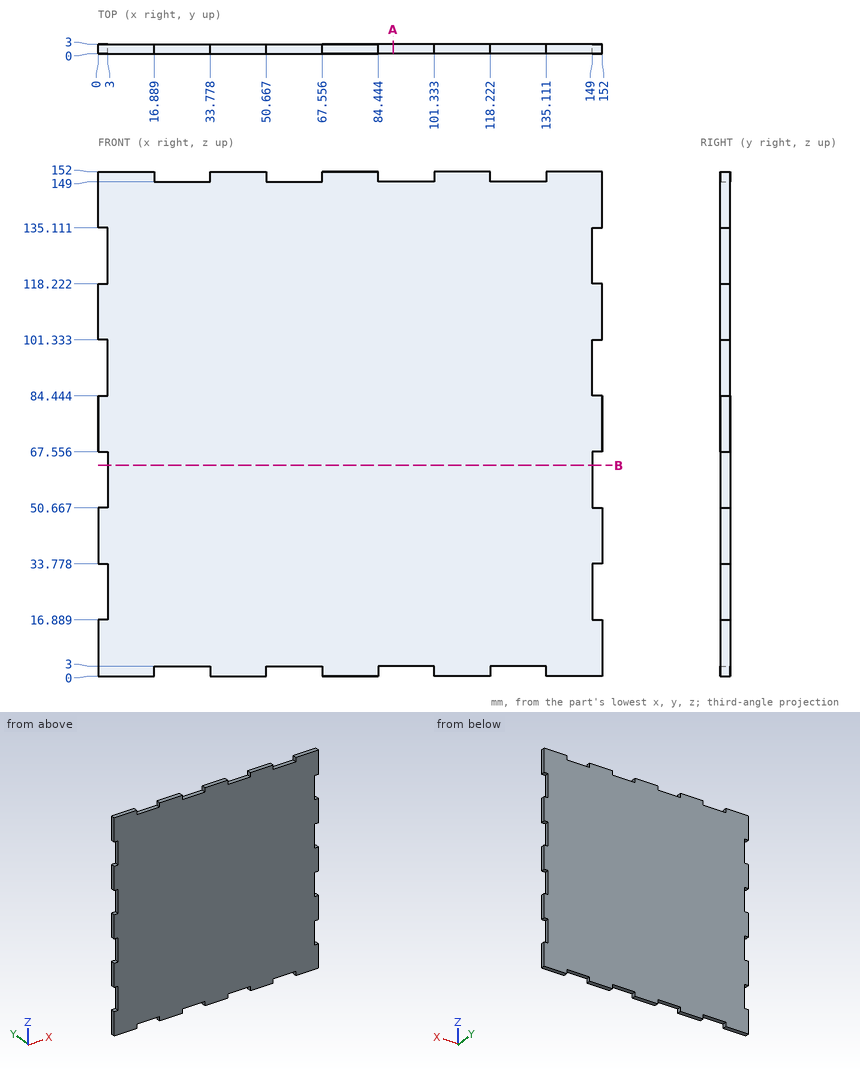
The drawing under review shows one solid part. Ordinate dimensions are in mm from its lowest x, y, z. Give positions to 0.01 mm unless a question says otherwise; leave off trailing zeros. Write each loop counter-clockwise with the first axis right and the second up, starting at its lowest first coordinate (ties: lowest second). Pieces come first, ordered by that corner, then holes. Notation, with made-up numbers: (35.5, 87) - (49.5, 87) arc R17 cw to (49.5, 98) - close; hole circle Ø8 at (70.25, 0). An arc over 180 degrees is marked (long way). Answer in a Markdown table with one row per item. Add a question column.
1. We need section B-B on z = 63.5. Write out the cut boundary in (x, y).
2. We need section A-A on x = 89. Write out the cut boundary in (y, z).
3. Wall thickness on line 1 along Z through (x, y) = (17, 0.2): over which ranges is the line inside the solid? List them lowest first. Write a range as [from, to].
4. Insertion check: P1, Ø0.9, axis at x = 128, y = 2, coming from the +Z side; P2, Ø2, axis at x = 80, z = 73, coming from the -Y side; P3, Ø1.5, axis at x = 89.5, y = 2, coming from the -Z side; P4, Ø1.5, axis at y = 0.5, z = 128, coming from the +X side. Each pin has a flat end and moves straight along its axis. Give the tip position at first contact, or say it passes through.
Ans:
| question | item | result |
|---|---|---|
| 1 | outline | (3, 0) - (149, 0) - (149, 3) - (3, 3) - close |
| 2 | outline | (0, 3) - (3, 3) - (3, 149) - (0, 149) - close |
| 3 | line 1 | z = [3, 149] |
| 4 | P1 | stops at z = 149 |
| 4 | P2 | stops at y = 0 |
| 4 | P3 | stops at z = 3 |
| 4 | P4 | stops at x = 149 |
